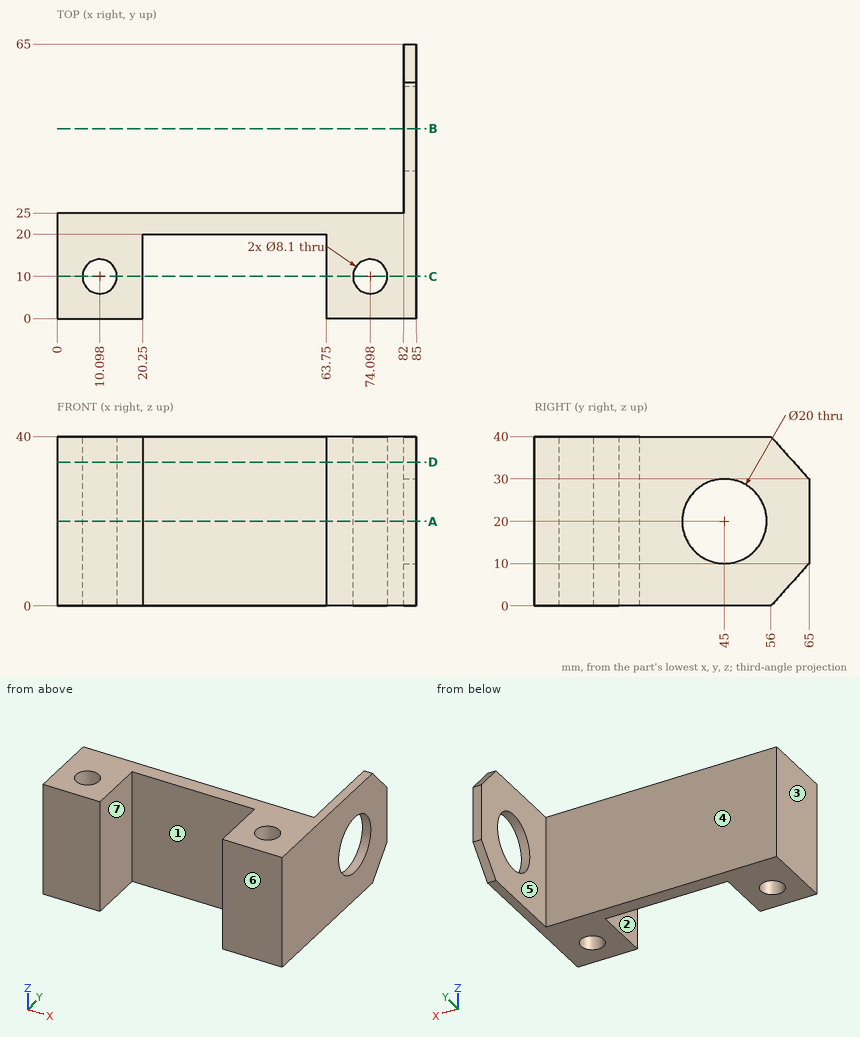
Geometry check sheet. Reference: drawing and pictorial views, mm from the part's lowest x, y, z. A direction names the side the tool comes from. Give positions to 0.01 mm unless a question says otherwise; leave off trailing zeros. Order: outer loops, then holes, each group sorted by start corner. A loop starts at its lowest first (then second) coordinate and runs counter-clockwise, first axis right, second up. Notation, with made-up numbers: M 52,31.5 L 61,31.5 A10 ccw 61,50.5 Z; hole C -36,41 d1. An arc over 180 degrees is marked long. Answer in a Markdown table with one row per item. Add a question column.
Item 1: Section check D-D, the plane z = 34. Enter the section's corners in (x, y), and give its area (3 significant figures).
Item 2: Tool access check on the marked faces 5, 6 and 7. Record the directions out of +Z, -Z, +X, -X, +Y, -Y that give a thin tool (end or side, any length) a straight path to the whole face; none if there is none.
Item 3: Section check B-B, the plane y = 45. Enter the section's corners in (x, z), and give its area (3 significant figures).
Item 4: Mould release check, pull along X, two halves, no side actions. Record for the marked faces 1, 2, 3 and 4: released by +X, released by -X, zero draft, split by the parting line, or undercut.
Item 5: Section check C-C, the plane y = 10. Enter the section's corners in (x, z), and give its area (3 significant figures).
Item 6: Gauge pin test, flat ends, axial feed: pin 1 (12 mm diameter, centred on y = 42.5, z = 6.5, fed in from -X); pin 2 (1 mm diameter, centred on y = 54, z = 20.5, fed in from +X); pin 3 (4 mm diameter, centred on x = 34, z = 15.5, fed in from -Y). Record the tip position at first contact, or that the pin passes through.
Item 7: Section check A-A, the plane z = 20. Enter the section's corners in (x, y).
Item 8: Scan lines: probe 1 along X at (y, z) = (16, 17); probe 2 along X at (y, z) = (8, 31.5); probe 3 along Y at (x, z) = (20, 11). Record each from-to range of solid material in increasing order. Write a range as from..to.
Filled sheet:
| question | item | result |
|---|---|---|
| 1 | outline | M 0,0 L 20.25,0 L 20.25,20 L 63.75,20 L 63.75,0 L 85,0 L 85,61.4 L 82,61.4 L 82,25 L 0,25 Z; hole C 10.1,10 d8.1; hole C 74.1,10 d8.1 |
| 1 | area | 1,260 mm^2 |
| 2 | face 5 | +Z, -Z, -X, +Y |
| 2 | face 6 | +Z, -Z, +X, -X, -Y |
| 2 | face 7 | +Z, -Z, -Y |
| 3 | outline | M 82,0 L 85,0 L 85,10 L 82,10 Z; M 82,30 L 85,30 L 85,40 L 82,40 Z |
| 3 | area | 60.0 mm^2 |
| 4 | face 1 | undercut |
| 4 | face 2 | undercut |
| 4 | face 3 | released by -X |
| 4 | face 4 | zero draft |
| 5 | outline | M 0,0 L 6.05,0 L 6.05,40 L 0,40 Z; M 14.15,0 L 20.25,0 L 20.25,40 L 14.15,40 Z; M 63.75,0 L 70.05,0 L 70.05,40 L 63.75,40 Z; M 78.15,0 L 85,0 L 85,40 L 78.15,40 Z |
| 5 | area | 1,010 mm^2 |
| 6 | pin 1 | stops at x = 82 |
| 6 | pin 2 | passes through |
| 6 | pin 3 | stops at y = 20 |
| 7 | outline | M 0,0 L 20.25,0 L 20.25,20 L 63.75,20 L 63.75,0 L 85,0 L 85,35 L 82,35 L 82,25 L 0,25 Z; M 82,55 L 85,55 L 85,65 L 82,65 Z; hole C 10.1,10 d8.1; hole C 74.1,10 d8.1 |
| 8 | probe 1 | x = 0..20.25, 63.75..85 |
| 8 | probe 2 | x = 0..6.58, 13.62..20.25, 63.75..70.58, 77.62..85 |
| 8 | probe 3 | y = 0..25 |
